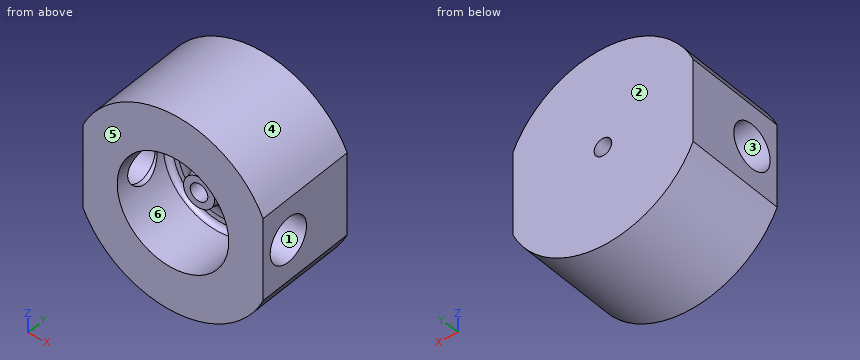
from build123d import *

# Parameters (mm, degrees)
F_1_4_28_TAPPED_HOLE1_D = 5.4102
SKETCH4_W               = 25.4
SKETCH4_H               = 25.4
FLATS_DEPTH             = 54.536186827
FILLET1_R               = 1.5875


with BuildPart() as part:
    # Sketch1 → Revolve1 (revolve)
    with BuildSketch(Plane.XY, mode=Mode.PRIVATE) as revolve1_sk:
        with BuildLine():
            Line((0, 31.75), (-30.48, 31.75))
            Line((-30.48, 31.75), (-30.48, 0))
            Line((-30.48, 0), (-17.145, 0))
            Line((-17.145, 0), (-17.145, 19.05))
            Line((-17.145, 19.05), (-13.97, 19.05))
            ThreePointArc((-13.97, 19.05), (-7.459314312, 16.353185688), (-4.7625, 9.8425))
            Line((-4.7625, 9.8425), (0, 9.8425))
            Line((0, 9.8425), (0, 31.75))
        make_face()
    revolve(revolve1_sk.sketch.rotate(Axis((0, 0, 0), (0, 1, 0)), 180), axis=Axis((0, 0, 0), (0, 1, 0)))

    # 1/4-28 Tapped Hole1 (through all)
    with Locations(Plane(origin=(0, 31.75, 0), x_dir=(1, 0, 0), z_dir=(0, 1, 0))):
        with Locations((0, 0)):
            Hole(F_1_4_28_TAPPED_HOLE1_D / 2)

    # Sketch4 → flats (cut, through all)
    with BuildSketch(Plane(origin=(0, 0, 0), x_dir=(1, 0, 0), z_dir=(0, 1, 0))):
        with Locations((-40.408128771, 0)):
            Rectangle(SKETCH4_W, SKETCH4_H)
        with Locations((40.408128771, 0)):
            Rectangle(SKETCH4_W, SKETCH4_H)
    extrude(amount=FLATS_DEPTH, mode=Mode.SUBTRACT)

    # Sketch6 → 1/4 NPT Tapped Hole1 (revolve, cut)
    with BuildSketch(Plane(origin=(27.708128771, 9.525, 0), x_dir=(0, 0, -1), z_dir=(0, 1, 0))):
        Polygon((0, 0), (0, 20.614347279), (5.5626, 17.272), (5.5626, 9.906), (6.557984794, 9.906), (6.8545837, 0), align=None)
    f_1_4_npt_tapped_hole1 = revolve(axis=Axis((34.058128771, 9.525, 0), (-1, 0, 0)), mode=Mode.SUBTRACT)

    # Mirror1: 1/4 NPT Tapped Hole1 across plane
    add(f_1_4_npt_tapped_hole1.mirror(Plane(origin=(0, 0, 0), x_dir=(0, 0, 1), z_dir=(1, 0, 0))), mode=Mode.SUBTRACT)

    # Fillet1
    fillet1_edges = [part.edges().sort_by_distance(p)[0] for p in [
        (-17.145, 19.05, 0),
    ]]
    fillet(fillet1_edges, radius=FILLET1_R)


solid = part.part
Read the model definition and answer for the solid it produces. Units are mm, in the model's axes. Face numbers are marked on the shaded views. A direction names the side the tool comes from. Coordinates: 2 decimals unless noted, no trailing zeros. Order: outer loops, then holes, each group sorted by start corner. A loop starts at its lowest first (then second) coordinate and runs counter-clockwise, first axis right, second up. Notation, with made-up numbers: M 60.25,-38.5 L 96.25,-38.5 A4 cw 96.25,-33.5 Z; hole C 50,73 d7. An arc over 180 degrees is marked long. Put each result on its own line as item: value. Start each with the question number.
Item 1: For the marked faces 5 and 6, determine the directions among +Z, -Z, +X, -X, +Y, -Y from which every point of the face is accessible in a straight line to the end or side of a thin tool.
Item 2: The mould has two halves that part along Y. Classify the marked faces 1, 2, 3 and 4: +Y half, -Y half, draft (parallel to the pull), parting line (faces both ways), or undercut.
Item 3: Section C-C, the plane y = 23 is taken. Determine the outline of the cut face in (x, z).
Item 4: Consider probe 1 along X at (y, z) = (17, 4.5); probe 2 along Z at (x, y) = (0, 13) (3 decimals); probe 3 along Z at (x, y) = (0, 7.25) (3 decimals). Determine where each line is inside the solid, lowest interval first. Write a range as [from, to].
Item 5: Section D-D, the plane x = -19.5 is taken. Determine the outline of the cut face in (y, z) (3 decimals).
Item 6: Section B-B, the plane z = 0 is taken. Count the separate pieces of the cut face and the enclosed holes in it, plus the area to 3 significant figures.
Item 7: Given pin 1 Ø9 at (y, z) = (9.525, 0) entering from +X; pin 2 Ø12 at (x, y) = (-1, 7.5) entering from +Z; pin 3 Ø1 at (y, z) = (26, -17.5) entering from +X, each flat-ended and moving along its own axis, determine where each tip first touches the part or whether it passes through.
Computed:
1. face 5: +Z, -Z, +X, -X, -Y
1. face 6: -Y
2. face 1: undercut
2. face 2: +Y half
2. face 3: undercut
2. face 4: draft
3. outline: M -27.71,-12.7 A30.48 ccw 27.71,-12.7 L 27.71,12.7 A30.48 ccw -27.71,12.7 Z; hole C 0,0 d5.41
4. probe 1: x = [-27.71, -16.54], [-6.83, 6.83], [16.54, 27.71]
4. probe 2: z = [-30.48, -17.145], [-5.321, -2.705], [2.705, 5.321], [17.145, 30.48]
4. probe 3: z = [-30.48, -17.145], [17.145, 30.48]
5. outline: M 0,-23.426 L 31.75,-23.426 L 31.75,23.426 L 0,23.426 Z; hole C 9.525,0 d13.218
6. separate pieces: 4
6. enclosed holes: 0
6. area: 833 mm2
7. pin 1: stops at x = 5.77
7. pin 2: stops at z = 30.48
7. pin 3: stops at x = 25.3
